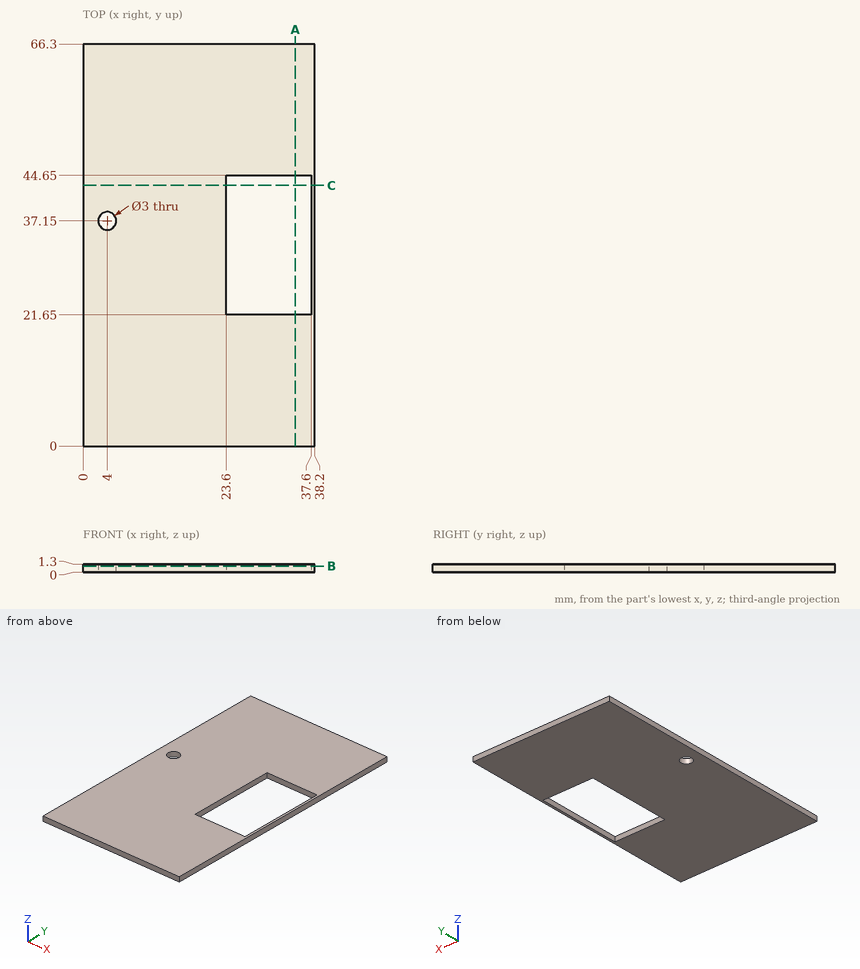
Answer from the drawing. Dimensions are ordinates in mm from the lowest x, y and z of the part. Coordinates: 2 decimals unless noted, no trailing zeros. Loops run counter-clockwise (first coordinate to the right, second up) from the corner with the lowest first, then second, coordinate; pieces in that order, holes last. Notation, with made-up numbers: (55, 65.25) - (82, 65.25) arc R22 ccw to (82, 75.25) - close; hole circle Ø11 at (-7, 84.5). An arc over 180 degrees is marked (long way). Use a Markdown table: item, result.
Item 1: Find section A-A, the plane x = 35. Determine the outline of the cut face in (y, z).
Evaluation:
| item | result |
|---|---|
| outline | (0, 0) - (21.65, 0) - (21.65, 1.3) - (0, 1.3) - close; (44.65, 0) - (66.3, 0) - (66.3, 1.3) - (44.65, 1.3) - close |
Item 2: Consider probe 1 along X at (y, z) = (37.15, 0.35); probe 2 along X at (y, z) = (22, 0.55); probe 3 along Y at (x, z) = (25, 0.9). Determine where each line is inside the solid, lowest interval first. Write a range as from..to.
Evaluation:
| item | result |
|---|---|
| probe 1 | x = 0..2.5, 5.5..23.6, 37.6..38.2 |
| probe 2 | x = 0..23.6, 37.6..38.2 |
| probe 3 | y = 0..21.65, 44.65..66.3 |
Item 3: Find section C-C, the plane y = 43. Determine the outline of the cut face in (x, z).
Evaluation:
| item | result |
|---|---|
| outline | (0, 0) - (23.6, 0) - (23.6, 1.3) - (0, 1.3) - close; (37.6, 0) - (38.2, 0) - (38.2, 1.3) - (37.6, 1.3) - close |
Item 4: Given pin 1 Ø5 at (x, y) = (4, 37.15) entering from -Z, flat-ended and moving along its own axis, determine where the tip first touches the part or whether it passes through.
Evaluation:
| item | result |
|---|---|
| pin 1 | stops at z = 0 |
Item 5: Find section B-B, the plane z = 1. Determine the outline of the cut face in (x, y), and give its area (3 significant figures).
Evaluation:
| item | result |
|---|---|
| outline | (0, 0) - (38.2, 0) - (38.2, 66.3) - (0, 66.3) - close; hole circle Ø3 at (4, 37.15); hole (23.6, 21.65) - (37.6, 21.65) - (37.6, 44.65) - (23.6, 44.65) - close |
| area | 2,200 mm2 |
